```python
from build123d import *

# Parameters (mm, degrees)
SKETCH1_W           = 44.45
SKETCH1_H           = 20.6375
BOSS_EXTRUDE1_DEPTH = 1.5875
SKETCH2_R           = 7.9375
BOSS_EXTRUDE2_DEPTH = 12.7
SKETCH3_W           = 9.525
SKETCH3_H           = 3.175
BOSS_EXTRUDE3_DEPTH = 3.175


with BuildPart() as part:
    # Sketch1 → Boss-Extrude1 (new body)
    with BuildSketch(Plane.XY):
        Rectangle(SKETCH1_W, SKETCH1_H)
    extrude(amount=BOSS_EXTRUDE1_DEPTH)

    # Sketch2 → Boss-Extrude2 (add)
    with BuildSketch(Plane.XY.offset(1.5875)):
        with Locations((-12.7, 0)):
            Circle(SKETCH2_R)
    boss_extrude2 = extrude(amount=BOSS_EXTRUDE2_DEPTH)

    # Mirror1: Boss-Extrude2 across plane
    add(boss_extrude2.mirror(Plane(origin=(0, 0, 0), x_dir=(0, 0, 1), z_dir=(1, 0, 0))))

    # Sketch3 → Boss-Extrude3 (add)
    with BuildSketch(Plane.XY.offset(1.5875)):
        with Locations((0, 7.750431081)):
            Rectangle(SKETCH3_W, SKETCH3_H)
    extrude(amount=BOSS_EXTRUDE3_DEPTH)


solid = part.part
```
For this review, take the finished solid that the model builds, in its own axes (mm). A direction names the side the tool comes from. Give positions to 0.01 mm unless a question says otherwise; leave off trailing zeros. Loops run counter-clockwise (first coordinate to the right, second up) from the corner with the lowest first, then second, coordinate; pieces in that order, holes last. Notation, with made-up numbers: M -2,62.5 L 6,62.5 A36 ccw 6,100.5 Z; hole C 2,59.25 d2. An arc over 180 degrees is marked long. One line per item, written item: value. Start each with the question number.
Q1. Add section A-A (z = 3). Give the boundary of the cut face in (x, y) (1 decimal), and give its area (3 significant figures).
Q2. Machinability: for faces 1 (the face through (0, 8, 4.762)), 2 (the face through (4.762, 8, 3)), 3 (the face through (0, 6.163, 3)), 4 (the face through (20.63, 0.35, 7.85)), 5 (the face through (0, 9.338, 3)), which of the approach directions +Z, -Z, +X, -X, +Y, -Y give a long, thin tool a straight path to every point of the face, cutting with its end or side? Answer none if there is none.
Q3. Draft analysis for pull direction X (two halves, no side actions). For faces 6 (the face through (0, 0, 0)), 7 (the face through (-22.225, 0, 1)), 8 (the face through (-4.762, 8, 3)), state which applies: released by +X, released by -X, zero draft, split by the parting line, or undercut.
Q4. Clearance check with flat-ended pins moving along their axes: pin 1 Ø4 at (x, y) = (4.5, -7) entering from +Z; pin 2 Ø1 at (x, z) = (10, 6) entering from +Y; pin 3 Ø1 at (y, z) = (-3.5, 6) entering from +X. State where each tip first meets the part, or that it passes through.
Q5. Add section D-D (z = 12.5). Give the boundary of the cut face in (x, y) (1 decimal), and give its area (3 significant figures).
Q6. Add section B-B (y = 0). Give the boundary of the cut face in (x, z) (1 decimal).
Q7. For L1, parallel to Z at x = -5, y = 3.25; L2, parallel to X at y = 2.5, z = 3.75; L3, parallel to Y at x = 2, z = 4, list the stretches that pass through material, from the lowest coordinate up.
Q8. Add section C-C (x = 12.7). Give the boundary of the cut face in (y, z), and give its area (3 significant figures).
Reply:
1. outline: C -12.7,0 d15.9; M -4.8,6.2 L 4.8,6.2 L 4.8,9.3 L -4.8,9.3 Z; C 12.7,0 d15.9
1. area: 426 mm²
2. face 1: +Z, +Y, -Y
2. face 2: +Z, +Y
2. face 3: +Z, -Y
2. face 4: +Z
2. face 5: +Z, +X, -X, +Y
3. face 6: zero draft
3. face 7: released by -X
3. face 8: undercut
4. pin 1: z = 1.59
4. pin 2: y = 7.63
4. pin 3: x = 20.05
5. outline: C -12.7,0 d15.9; C 12.7,0 d15.9
5. area: 396 mm²
6. outline: M -22.2,0 L 22.2,0 L 22.2,1.6 L 20.6,1.6 L 20.6,14.3 L 4.8,14.3 L 4.8,1.6 L -4.8,1.6 L -4.8,14.3 L -20.6,14.3 L -20.6,1.6 L -22.2,1.6 Z
7. L1: 0 to 1.59
7. L2: -20.23 to -5.17, 5.17 to 20.23
7. L3: 6.16 to 9.34
8. outline: M -10.32,0 L 10.32,0 L 10.32,1.59 L 7.94,1.59 L 7.94,14.29 L -7.94,14.29 L -7.94,1.59 L -10.32,1.59 Z
8. area: 234 mm²
